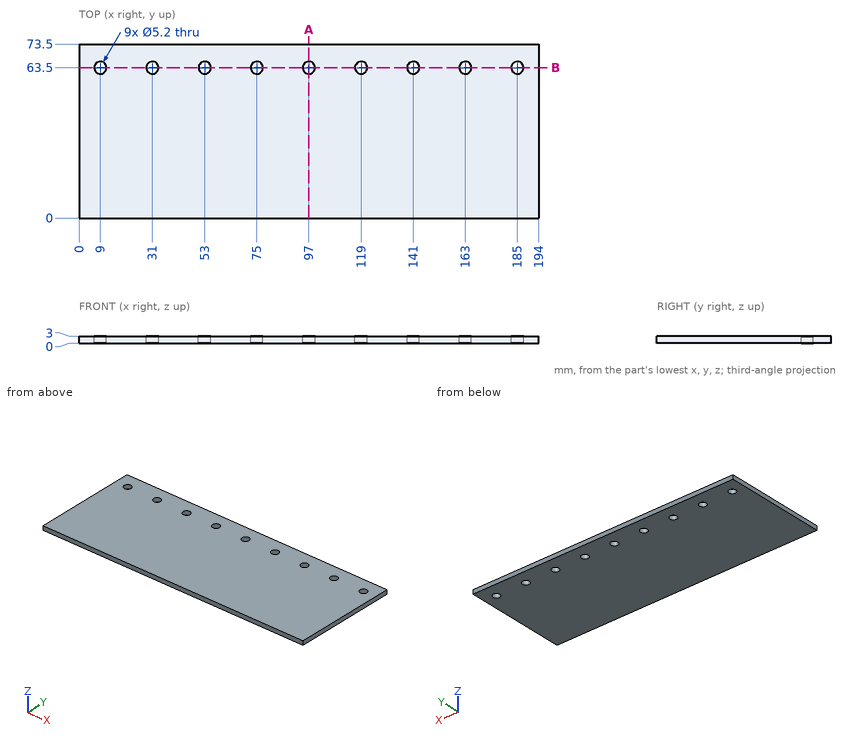
Geometry check sheet. Reference: drawing and pictorial views, mm from the part's lowest x, y, z. Round coordinates to 2 decimals unless told otherwise and drop trailing zeros. Write each loop counter-clockwise with the first axis right and the second up, starting at its lowest first coordinate (ties: lowest second). Pieces come first, ordered by that corner, then holes.
Item 1: Material ranges on line 1 along Y through (x, z) = (53, 1.75), recorded low to high.
Determined:
line 1: y = 0 to 60.9, 66.1 to 73.5
Item 2: Section check B-B (y = 63.5). Give the number of separate pieces and of enclosed holes in the cut face, plus the area to 3 significant figures.
Determined:
separate pieces: 10
enclosed holes: 0
area: 442 mm2
Item 3: Section check A-A (x = 97). Record the boundary of the cut face in (y, z).
Determined:
outline: (0, 0) - (60.9, 0) - (60.9, 3) - (0, 3) - close; (66.1, 0) - (73.5, 0) - (73.5, 3) - (66.1, 3) - close
Item 4: Go/stop test with a flat-tipped pin: pin 1 Ø4.5 at (x, y) = (141, 63.5) entering from +Z. Record where the tip stops, or that it passes through.
Determined:
pin 1: passes through
